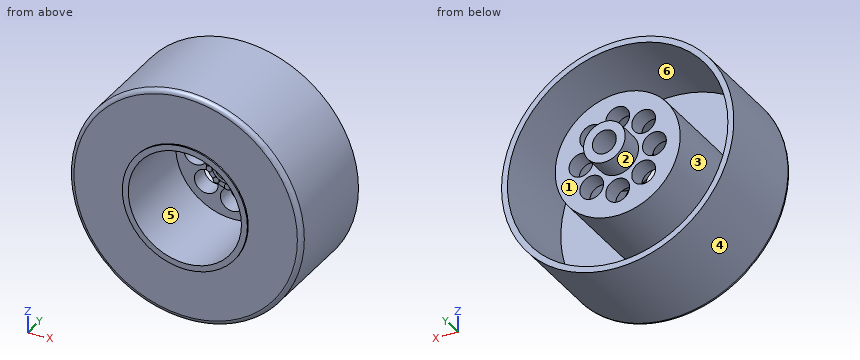
from build123d import *
from build123d import SkipClean  # not in build123d's __all__

# Parameters (mm, degrees)
F0_R      = 19.5
F1_DEPTH  = 17
F2_R      = 9.5
F3_DEPTH  = 14
F4_R      = 18.5
F4_R_2    = 10.5
F5_DEPTH  = 16
F6_R      = 2
F7_DEPTH  = 25
F8_R      = 3.5
F9_DEPTH  = 4
F10_R     = 2
F11_DEPTH = 138.7
F12_R     = 4
F12_R_2   = 2
F13_DEPTH = 1
F14_R     = 2.5
F14_R_2   = 2
F15_DEPTH = 0.75
F16_R     = 0.5
F17_DEPTH = 0.5
F19_R     = 0.75
F18_R     = 10.5
F18_R_2   = 9.5
F20_DEPTH = 0.25


# Not quite as in the source:
# - after a boolean that leaves OpenCascade's solid faulty, fix() repairs it


with BuildPart() as f1:
    # F0 (on Front) → F1 (new body)
    with BuildSketch(Plane.XZ):
        Circle(F0_R)
    extrude(amount=F1_DEPTH)

    # F2 (on face) → F3 (cut)
    with BuildSketch(Plane.XZ.offset(17)):
        Circle(F2_R)
    extrude(amount=-F3_DEPTH, mode=Mode.SUBTRACT)

    # F4 (on face) → F5 (cut)
    with BuildSketch(Plane(origin=(0, 0, 0), x_dir=(-1, 0, 0), z_dir=(0, 1, 0))):
        Circle(F4_R)
        Circle(F4_R_2, mode=Mode.SUBTRACT)
    extrude(amount=-F5_DEPTH, mode=Mode.SUBTRACT)

    # F6 (on face) → F7 (cut)
    with BuildSketch(Plane.XZ.offset(3)):
        with Locations((0, 6.1688632704)):
            Circle(F6_R)
        with Locations((-4.3620450507, 4.3620450507)):
            Circle(F6_R)
        with Locations((-6.1688632704, 0)):
            Circle(F6_R)
        with Locations((-4.3620450507, -4.3620450507)):
            Circle(F6_R)
        with Locations((0, -6.1688632704)):
            Circle(F6_R)
        with Locations((4.3620450507, -4.3620450507)):
            Circle(F6_R)
        with Locations((6.1688632704, 0)):
            Circle(F6_R)
        with Locations((4.3620450507, 4.3620450507)):
            Circle(F6_R)
    extrude(amount=-F7_DEPTH, mode=Mode.SUBTRACT)

    # F8 (on face) → F9 (join)
    with BuildSketch(Plane(origin=(0, 0, 0), x_dir=(-1, 0, 0), z_dir=(0, 1, 0))):
        Circle(F8_R)
    extrude(amount=F9_DEPTH)

    # F10 (on face) → F11 (cut)
    with BuildSketch(Plane(origin=(0, 4, 0), x_dir=(-1, 0, 0), z_dir=(0, 1, 0))):
        Circle(F10_R)
    extrude(amount=-F11_DEPTH, mode=Mode.SUBTRACT)

    # F12 (on face) → F13 (join)
    with BuildSketch(Plane.XZ.offset(3)):
        with Locations((0.0866679911, 0.0506265242)):
            Circle(F12_R)
        Circle(F12_R_2, mode=Mode.SUBTRACT)
    with SkipClean():  # cleaning this boolean's faces spoils the solid; the shape is the same uncleaned
        extrude(amount=F13_DEPTH)

    # F14 (on face) → F15 (join)
    with BuildSketch(Plane.XZ.offset(4)):
        Circle(F14_R)
        Circle(F14_R_2, mode=Mode.SUBTRACT)
    extrude(amount=F15_DEPTH)

    add(f1.part.fix(), mode=Mode.REPLACE)

    # F16 (on face) → F17 (join)
    with BuildSketch(Plane.XZ.offset(4)):
        with Locations((0, 3.2079922967)):
            Circle(F16_R)
        with Locations((-1.8856105614, 2.5953202858)):
            Circle(F16_R)
        with Locations((-3.050981978, 0.9913241375)):
            Circle(F16_R)
        with Locations((-3.050981978, -0.9913241375)):
            Circle(F16_R)
        with Locations((-1.8856105614, -2.5953202858)):
            Circle(F16_R)
        with Locations((0, -3.2079922967)):
            Circle(F16_R)
        with Locations((1.8856105614, -2.5953202858)):
            Circle(F16_R)
        with Locations((3.050981978, -0.9913241375)):
            Circle(F16_R)
        with Locations((3.050981978, 0.9913241375)):
            Circle(F16_R)
        with Locations((1.8856105614, 2.5953202858)):
            Circle(F16_R)
    extrude(amount=F17_DEPTH)

    # F19
    f19_edges = [f1.edges().sort_by_distance(p)[0] for p in [
        (-19.5, -17, 0),
    ]]
    fillet(f19_edges, radius=F19_R)

    # F18 (on face) → F20 (join)
    with BuildSketch(Plane.XZ.offset(17)):
        Circle(F18_R)
        Circle(F18_R_2, mode=Mode.SUBTRACT)
    extrude(amount=F20_DEPTH)


solid = f1.part
The model under review builds one solid part; all positions refer to its coordinate system, in mm. Face numbers are marked on the shaded views. A direction names the side the tool comes from. Round coordinates to 2 decimals unless told otherwise and drop trailing zeros. Loops run counter-clockwise (first coordinate to the right, second up) from the corner with the lowest first, then second, coordinate; pieces in that order, holes last. Notation, with made-up numbers: M 0,63 L 42,63 A24 ccw 42,89 Z; hole C -14.75,-13 d4. An arc over 180 degrees is marked long. Answer as a JSON object with one key per item and string values.
Item 1: Clearance check with flat-ended pins moving along their axes: P1, Ø0.8, axis at x = 3, z = 1, coming from the -Y side; P2, Ø10, axis at x = 7, y = -5.5, coming from the +Z side; P3, Ø2.5, axis at x = 0, z = 0, coming from the -Y side; P4, Ø3, axis at x = -11, z = -9, coming from the -Y side. State where each tip first meets the part, or that it passes through.
Check sheet entries:
{"P1": "y = -4.5", "P2": "z = 19.4", "P3": "through", "P4": "y = -17"}
Item 2: The part is to be moulded in two halves that separate along Z. For the marked faces 1, 2 and 3, say which applies: +Z half, -Z half, draft (parallel to the pull), parting line (faces both ways), or undercut.
Check sheet entries:
{"face 1": "draft", "face 2": "parting line", "face 3": "undercut"}
Item 3: We need section A-A, the plane y = -2.5. State how many separate pieces and enclosed holes the cut face has, and give its area (3 significant figures).
Check sheet entries:
{"separate pieces": "2", "enclosed holes": "10", "area": "353 mm2"}
Item 4: We need section B-B, the plane y = -7. State the section outline as (x, z) points, and give its area (3 significant figures).
Check sheet entries:
{"outline": "C 0,0 d39; C 0,0 d21; hole C 0,0 d37; hole C 0,0 d19", "area": "182 mm2"}
Item 5: For line 1 along Z through (x, y) = (0, -1.6); line 2 along X through (y, z) = (-7.25, -0.5); line 3 along X through (y, z) = (-5.25, -4), list the stretches that pass through material, from the lowest coordinate up.
Check sheet entries:
{"line 1": "-19.5 to -18.5, -10.5 to -8.17, -4.17 to -2, 2 to 4.17, 8.17 to 10.5, 18.5 to 19.5", "line 2": "-19.49 to -18.49, -10.49 to -9.49, 9.49 to 10.49, 18.49 to 19.49", "line 3": "-19.09 to -18.06, -9.71 to -8.62, 8.62 to 9.71, 18.06 to 19.09"}
Item 6: Tool access review of the marked faces 4, 5 and 6: name each direction out of +Z, -Z, +X, -X, +Y, -Y from which nothing blocks a thin tool from reaching the whole face with its end or side.
Check sheet entries:
{"face 4": "+Y, -Y", "face 5": "-Y", "face 6": "+Y"}
